Verification items for the finished model (mm, model axes). A direction names the side the tool comes from. Coordinates: 2 decimals unless noted, no trailing zeros. Write item = value, one per line. Start each with the question number.
(1) Gauge pin test, flat ends, axial feed: pin 1 Ø1 at (x, y) = (-3.5, 6) entering from -Z; pin 2 Ø1.5 at (x, z) = (4.5, 30.5) entering from -Y; pin 3 Ø2 at (x, z) = (3, 34.5) entering from -Y. Record the tip position at first contact, or that the pin passes through.
(2) Set-up check for faces 1 (the face through (5, -7.84, 36.13)), 2 (the face through (3.48, -1.1, 76.94)): record each of +Z, -Z, +X, -X, +Y, -Y from which the full face is reachable in a straight line by a thin tool's end or side.
(3) Material ranges on probe 1 along Z at (x, y) = (3, -3.5); probe 2 along X at (y, z) = (4.5, 14); probe 3 along Z at (x, y) = (1.5, 3), recorded low to high. Write a range as [from, to].
Autodesk Inventor part; units mm, degrees
ref_plane "YZ Plane" through (0, 0, 0) normal (1, 0, 0) x (0, 1, 0)
ref_plane "XZ Plane" through (0, 0, 0) normal (0, 1, 0) x (-1, 0, 0)
ref_plane "XY Plane" through (0, 0, 0) normal (0, 0, 1) x (1, 0, 0)
sketch "Sketch1" plane through (0, 0, 0) normal (0, 0, 1) x (1, 0, 0)
  circle A0 centre (0, 0) radius 9.3
  dimension "d0" = 18.6
extrude "Extrusion1" add sketch "Sketch1" along normal blind 73
sketch "Sketch2" plane through (0, 0, 73) normal (0, 0, 1) x (1, 0, 0)
  circle A0 centre (0, 0) radius 3.65
  dimension "d3" = 7.3
extrude "Extrusion2" add sketch "Sketch2" along normal blind 10
fillet "Fillet1" radius 6.7625 1 edges at (-9.3, 0, 73)
fillet "Fillet2" radius 2 1 edges at (-3.65, 0, 83)
fillet "Fillet3" radius 6.7625 1 edges at (-9.3, 0, 0)
properties part number "12g_CO2_Cartridge"
Response:
q1.pin_1 = 1.24
q1.pin_2 = -8.51
q1.pin_3 = -9.08
q2.face_1 = +Z, -Z
q2.face_2 = +Z
q3.probe_1 = [0.33, 72.77]
q3.probe_2 = [-8.14, 8.14]
q3.probe_3 = [0.05, 82.05]
